Part model, mm, in its own coordinate system. Give positions to 0.01 mm unless a question says otherwise; leave off trailing zeros. Write each loop counter-clockwise with the first axis right and the second up, starting at its lowest first coordinate (ties: lowest second). Pieces come first, ordered by that corner, then holes. Notation, with made-up numbers: M -31,-13 L 9,-13 A24 ccw 9,2 Z; hole C -33.5,-40 d5. An arc over 180 degrees is marked long. Use a Markdown table: item, result.
```python
from build123d import *

# Parameters (mm, degrees)
SKETCH1_R               = 5
BOSS_EXTRUDE1_DEPTH     = 326
CUT_EXTRUDE1_REACH      = 329.721
CUT_EXTRUDE1_END_RADIUS = 5
SKETCH2_R               = 3.3234375


with BuildPart() as part:
    # Sketch1 → Boss-Extrude1 (new body)
    with BuildSketch(Plane(origin=(0, 0, 0), x_dir=(1, 0, 0), z_dir=(0, 1, 0))):
        with BuildLine():
            Line((4.191872704, 5.606086267), (11.5870568, 13.001270363))
            Line((11.5870568, 13.001270363), (4.001270363, 13.001270363))
            Line((4.001270363, 13.001270363), (4.001270363, 15.001270363))
            Line((4.001270363, 15.001270363), (15.001270363, 15.001270363))
            Line((15.001270363, 15.001270363), (15.001270363, 4.001270363))
            Line((15.001270363, 4.001270363), (13.001270363, 4.001270363))
            Line((13.001270363, 4.001270363), (13.001270363, 11.5870568))
            Line((13.001270363, 11.5870568), (5.606086267, 4.191872704))
            ThreePointArc((5.606086267, 4.191872704), (7, 0), (5.606086267, -4.191872704))
            Line((5.606086267, -4.191872704), (13.001270363, -11.5870568))
            Line((13.001270363, -11.5870568), (13.001270363, -4.001270363))
            Line((13.001270363, -4.001270363), (15.001270363, -4.001270363))
            Line((15.001270363, -4.001270363), (15.001270363, -15.001270363))
            Line((15.001270363, -15.001270363), (4.001270363, -15.001270363))
            Line((4.001270363, -15.001270363), (4.001270363, -13.001270363))
            Line((4.001270363, -13.001270363), (11.5870568, -13.001270363))
            Line((11.5870568, -13.001270363), (4.191872704, -5.606086267))
            ThreePointArc((4.191872704, -5.606086267), (0, -7), (-4.191872704, -5.606086267))
            Line((-4.191872704, -5.606086267), (-11.5870568, -13.001270363))
            Line((-11.5870568, -13.001270363), (-4.001270363, -13.001270363))
            Line((-4.001270363, -13.001270363), (-4.001270363, -15.001270363))
            Line((-4.001270363, -15.001270363), (-15.001270363, -15.001270363))
            Line((-15.001270363, -15.001270363), (-15.001270363, -4.001270363))
            Line((-15.001270363, -4.001270363), (-13.001270363, -4.001270363))
            Line((-13.001270363, -4.001270363), (-13.001270363, -11.5870568))
            Line((-13.001270363, -11.5870568), (-5.606086267, -4.191872704))
            ThreePointArc((-5.606086267, -4.191872704), (-7, 0), (-5.606086267, 4.191872704))
            Line((-5.606086267, 4.191872704), (-13.001270363, 11.5870568))
            Line((-13.001270363, 11.5870568), (-13.001270363, 4.001270363))
            Line((-13.001270363, 4.001270363), (-15.001270363, 4.001270363))
            Line((-15.001270363, 4.001270363), (-15.001270363, 15.001270363))
            Line((-15.001270363, 15.001270363), (-4.001270363, 15.001270363))
            Line((-4.001270363, 15.001270363), (-4.001270363, 13.001270363))
            Line((-4.001270363, 13.001270363), (-11.5870568, 13.001270363))
            Line((-11.5870568, 13.001270363), (-4.191872704, 5.606086267))
            ThreePointArc((-4.191872704, 5.606086267), (0, 7), (4.191872704, 5.606086267))
        make_face()
        with Locations(Location((0, 0, 0), (0, 0, 270))):
            Circle(SKETCH1_R, mode=Mode.SUBTRACT)
    extrude(amount=BOSS_EXTRUDE1_DEPTH)

    # Cut-Extrude1: up to this cylinder (the profile starts outside it)
    cut_extrude1_end = Plane(origin=(0, 82, 0), z_dir=(0, -1, 0)) * Cylinder(CUT_EXTRUDE1_END_RADIUS, 670.442, mode=Mode.PRIVATE)
    # Sketch2 → Cut-Extrude1 (cut, up to the surface)
    with BuildSketch(Plane.XY.offset(15.001270363), mode=Mode.PRIVATE) as cut_extrude1_sk1:
        with Locations((-0.001270363, 82)):
            Circle(SKETCH2_R)
    cut_extrude1_tool1 = extrude(cut_extrude1_sk1.sketch, amount=-CUT_EXTRUDE1_REACH, mode=Mode.PRIVATE) - cut_extrude1_end
    add(cut_extrude1_tool1.solids().sort_by_distance((-0.00127, 82, 15.00127))[0], mode=Mode.SUBTRACT)


solid = part.part
```
1. Cut at B-B, the plane x = 0. Give the cut face in (y, z).
Findings below:
| item | result |
|---|---|
| outline | M 0,-7 L 326,-7 L 326,-5 L 0,-5 Z; M 0,5 L 78.68,5 L 78.68,7 L 0,7 Z; M 85.32,5 L 326,5 L 326,7 L 85.32,7 Z |
2. Two-plate mould, pull along X, no slides. Class faces 1 (the flat face through (-15.001, 161, 10)), 2 (the flat face through (-7.838, 160.718, 9.252)), 3 (the flat face through (-9, 161, 15.001)): released by +X, released by -X, zero draft, split by the parting line, or undercut.
Findings below:
| item | result |
|---|---|
| face 1 | released by -X |
| face 2 | undercut |
| face 3 | zero draft |
3. Drill centre lines: L1, parallel to X at y = 235, z = 0; L2, parallel to Z at x = 7.5, y = 237.5; L3, parallel to X at y = 229, z = -8.5. Where is each one in solid material? Low to high.
Findings below:
| item | result |
|---|---|
| L1 | -7 to -5, 5 to 7 |
| L2 | -15 to -13, -8.91 to -6.09, 6.09 to 8.91, 13 to 15 |
| L3 | -15 to -13, -9.91 to -7.09, 7.09 to 9.91, 13 to 15 |
4. Drop flat-ended pins along their axis: P1, Ø4, axis at x = 0, y = 82, coming from the -Z side; P2, Ø12, axis at y = 251.5, z = -1, coming from the +X side. Give the stop position or say it passes through.
Findings below:
| item | result |
|---|---|
| P1 | z = -7 |
| P2 | x = 15 |
5. Cut at A-A, the plane z = 0. Give the cut face in (x, y).
Findings below:
| item | result |
|---|---|
| outline | M -7,0 L -5,0 L -5,326 L -7,326 Z; M 5,0 L 7,0 L 7,326 L 5,326 Z |
